Check sheet for the modelled part. Datum: model origin and axes. Units: mm. A direction names the side the tool comes from. Give positions to 0.01 mm unless a question says otherwise; leave off trailing zeros. Loops run counter-clockwise (first coordinate to the right, second up) from the corner with the lowest first, then second, coordinate; pieces in that order, holes last. Notation, with made-up numbers: (-5, -5.5) - (32, -5.5) arc R19 cw to (32, 22.5) - close; hole circle Ø6 at (88.5, -34). An arc over 180 degrees is marked (long way). Use one line per item in the form item = value.
from build123d import *

# Parameters (mm, degrees)
F0_R            = 30
F0_R_2          = 10
F1_DEPTH        = 10
F2_R            = 15
F2_R_2          = 10
F3_DEPTH        = 10
F4_R            = 4
F5_DEPTH        = 10.001
F5_COPIES_COUNT = 6


# Not quite as in the source:
# - a pattern or mirror of a feature is missing from the dataset's text; its kind, count and spacing are read off the source's solid


with BuildPart() as f1:
    # F0 (on Top) → F1 (new body)
    with BuildSketch(Plane.XY):
        Circle(F0_R)
        Circle(F0_R_2, mode=Mode.SUBTRACT)
    extrude(amount=F1_DEPTH)

    # F2 (on face) → F3 (join)
    with BuildSketch(Plane.XY.offset(10)):
        Circle(F2_R)
        Circle(F2_R_2, mode=Mode.SUBTRACT)
    extrude(amount=F3_DEPTH)

    # F4 (on face) → F5 (cut, through all)
    with BuildSketch(Plane.XY.offset(10)):
        with Locations((0, 22.5)):
            Circle(F4_R)
    f5 = extrude(amount=-F5_DEPTH, mode=Mode.SUBTRACT)

    # F5_copies: F5 ×6 about axis
    f5_copies_axis = Axis((0, 0, 0), (0, 0, 1))
    for i in range(1, F5_COPIES_COUNT):
        add(f5.rotate(f5_copies_axis, i * 360 / F5_COPIES_COUNT), mode=Mode.SUBTRACT)


solid = f1.part
Item 1: Section check C-C on x = -5. Record the boundary of the cut face in (y, z).
Answer block:
outline = (-29.58, 0) - (-8.66, 0) - (-8.66, 20) - (-14.14, 20) - (-14.14, 10) - (-29.58, 10) - close; (8.66, 0) - (29.58, 0) - (29.58, 10) - (14.14, 10) - (14.14, 20) - (8.66, 20) - close
Item 2: Mould release check, pull along X, two halves, no side actions. Record for faces 1 (the face through (-14.985, 0.66, 14.93)), 2 (the face through (3, -10, 20)), 3 (the face through (-15.8, -12.8, 5.1)): released by +X, released by -X, zero draft, split by the parting line, or undercut.
Answer block:
face_1 = split by the parting line
face_2 = zero draft
face_3 = undercut
Item 3: Access from +Z, -Z, +X, -X, +Y, -Y to the whole of each face (thin tool, end or side, straight path). Record for faces 4 (the face through (6, 14, 10)), 5 (the face through (-18.965, 7.284, 5.07)).
Answer block:
face_4 = +Z
face_5 = +Z, -Z
Item 4: Thickness scan on L1, parallel to Y at x = 22, z = 2.25; L2, parallel to Y at x = 2.5, z = 2.5; L3, parallel to X at y = -12.5, z = 8.5. Record the ranges inside material, lowest first.
Answer block:
L1 = -20.4 to -14.36, -8.14 to 8.14, 14.36 to 20.4
L2 = -29.9 to -25.62, -19.38 to -9.68, 9.68 to 19.38, 25.62 to 29.9
L3 = -27.27 to -23.29, -15.69 to 15.69, 23.29 to 27.27
Item 5: Section check B-B on y = 11.25. Record the boundary of the cut face in (x, z).
Answer block:
outline = (-27.81, 0) - (-23.49, 0) - (-23.49, 10) - (-27.81, 10) - close; (-15.49, 0) - (15.49, 0) - (15.49, 10) - (9.92, 10) - (9.92, 20) - (-9.92, 20) - (-9.92, 10) - (-15.49, 10) - close; (23.49, 0) - (27.81, 0) - (27.81, 10) - (23.49, 10) - close
Item 6: Section check A-A on y = 0. Record the boundary of the cut face in (x, z), then the cut area to 3 significant figures.
Answer block:
outline = (-30, 0) - (-10, 0) - (-10, 20) - (-15, 20) - (-15, 10) - (-30, 10) - close; (10, 0) - (30, 0) - (30, 10) - (15, 10) - (15, 20) - (10, 20) - close
area = 500 mm2
Item 7: Gauge pin test, flat ends, axial feed: P1, Ø7, axis at x = 0, y = -22.5, coming from the +Z side; P2, Ø12, axis at x = -9.5, z = 6.5, coming from the -Y side; P3, Ø10, axis at x = 17.5, z = 14.5, coming from the +Y side; P4, Ø2, axis at y = -3.5, z = 10.5, coming from the +X side. Record the tip position at first contact, or that the pin passes through.
Answer block:
P1 = through
P2 = -29.8
P3 = 25.79
P4 = 29.88
Item 8: Section check D-D on z = 4. Record the boundary of the cut face in (x, y), then the cut area to 3 significant figures.
Answer block:
outline = circle Ø60 at (0, 0); hole circle Ø8 at (-19.49, -11.25); hole circle Ø8 at (-19.49, 11.25); hole circle Ø20 at (0, 0); hole circle Ø8 at (0, -22.5); hole circle Ø8 at (0, 22.5); hole circle Ø8 at (19.49, -11.25); hole circle Ø8 at (19.49, 11.25)
area = 2,210 mm2
